Could you check a few things on this drawing? It's one solid part, dimensions in mm from its lowest x, y, z. Give positions to 0.01 mm unless a question says otherwise; leave off trailing zeros. Write each loop counter-clockwise with the first axis right and the second up, starting at its lowest first coordinate (ties: lowest second). Pieces come first, ordered by that corner, then holes. Notation, with made-up numbers: (-8.75, 52.5) -> (-2.75, 52.5) arc R15 cw to (-2.75, 76.5) -> close; hole circle Ø7 at (-16, -29). An arc over 180 degrees is marked (long way). Answer as CSV lines item,"result". Start each with the question number.
1. If we section it at C-C on y = 2.55: Count the separate pieces of the cut face and the enclosed holes in it, plus the area to 3 significant figures.
2. If we mould it in two halves opening along X, with no side actions, what happens to the marked faces 1 and 2? For each: pulls with the +X half, pulls with the -X half, needs draft (parallel to the pull), parting line crosses it, or undercut.
3. If we section it at A-A on z = 30: Write out the boundary of the cut face in (x, y), plus the area to 3 significant figures.
4. I need wall thicknesses on line 1 (X direction, y = 0.25, z = 12); line 2 (Z direction, x = 37, y = 0.6); line 3 (X direction, y = 1.7, z = 14) (1 decimal). Which ranges of each line are inside material? Lowest first, please. Write a range as [from, to].
5. If we section it at B-B on x = 53: Write out the boundary of the cut face in (y, z).
6. I'm going to push flat-ended pins straight in: P1, Ø1.5, axis at y = 1, z = 15, coming from the -X side; P2, Ø0.9, axis at x = 18, y = 1.5, coming from the -Z side; P3, Ø1, axis at y = 2.5, z = 15, coming from the +X side; P4, Ø1.8, axis at x = 30, z = 30, coming from the -Y side. Where does each tip first touch, or does it pass through?
7. If we section it at D-D on x = 7.5: Write out the boundary of the cut face in (y, z).
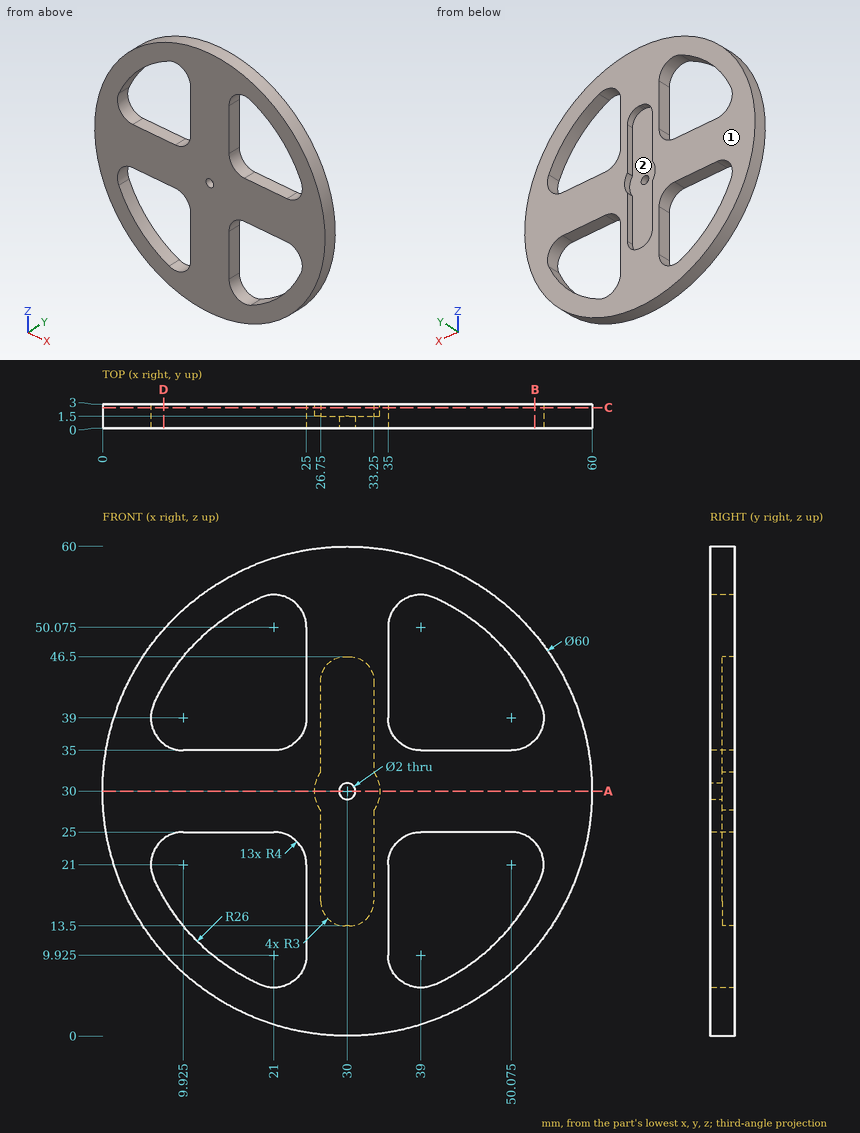
Computed values:
1,separate pieces,"1"
1,enclosed holes,"5"
1,area,"1,500 mm2"
2,face 1,"needs draft"
2,face 2,"undercut"
3,outline,"(0, 0) -> (29, 0) -> (29, 1.5) -> (26, 1.5) -> (26, 3) -> (0, 3) -> close; (31, 0) -> (60, 0) -> (60, 3) -> (34, 3) -> (34, 1.5) -> (31, 1.5) -> close"
3,area,"165 mm2"
4,line 1,"x = [6, 11.24], [25, 35], [48.76, 54]"
4,line 2,"z = [0.83, 6.46], [24.46, 35.54], [53.54, 59.17]"
4,line 3,"x = [4.6, 9.5], [25, 28.1], [31.9, 35], [50.5, 55.4]"
5,outline,"(0, 10.74) -> (3, 10.74) -> (3, 17.88) -> (0, 17.88) -> close; (0, 23.73) -> (3, 23.73) -> (3, 36.27) -> (0, 36.27) -> close; (0, 42.12) -> (3, 42.12) -> (3, 49.26) -> (0, 49.26) -> close"
6,P1,"stops at x = 3.6"
6,P2,"stops at z = 2.31"
6,P3,"stops at x = 56.26"
6,P4,"passes through"
7,outline,"(0, 10.16) -> (3, 10.16) -> (3, 16.97) -> (0, 16.97) -> close; (0, 24.18) -> (3, 24.18) -> (3, 35.82) -> (0, 35.82) -> close; (0, 43.03) -> (3, 43.03) -> (3, 49.84) -> (0, 49.84) -> close"
